Source: CAD feature listing. Evaluate the final solid. Frame: model axes, mm. A direction names the side the tool comes from. Round coordinates to 2 decimals unless told otherwise and drop trailing zeros. Order: outer loops, then holes, each group sorted by start corner. A loop starts at its lowest first (then second) coordinate and runs counter-clockwise, first axis right, second up. Notation, with made-up numbers: (62, 6.5) -> (77, 6.5) arc R29 cw to (77, 44.5) -> close; hole circle Ø4 at (62, 23.25). An arc over 180 degrees is marked (long way). Write item = value, one per line. Start each with the question number.
(1) Reachability of faces 1 (the face through (-26.959, -3.989, 4.068)), 2 (the face through (-102.128, -75, 50)) from +Z, -Z, +X, -X, +Y, -Y: full face, straight path, thin tool, end or side. Return the list, or none.
(2) Ray query, line 1 (X direction, y = -47, z = 56); line 2 (Y direction, x = -47.5, z = 81.5); line 3 (Z direction, x = -49, y = -128). Return the intervals inside material, ascending.
(3) Cut plane B-B on y = -57. Return the cut outline in (x, z).
(4) Cut plane C-C on x = 36. Return the cut outline in (y, z), then the cut area to 3 significant figures.
(5) Cut plane A-A on z = 40. Return the cut outline in (x, y).
from build123d import *

# Parameters (mm, degrees)
F0_W         = 152.4
F0_H         = 101.6
F1_DEPTH     = 152.4
F2_T         = -2.54
F3_T1_DEPTH  = 147.32
F3_T3_DEPTH  = 147.32
F3_T5_DEPTH  = 147.32
F3_T7_DEPTH  = 147.32
F3_T13_DEPTH = 160.02
F3_T19_DEPTH = 160.02
F3_T28_DEPTH = 160.02
F3_T34_DEPTH = 160.02
F3_T43_DEPTH = 160.02
F3_T49_DEPTH = 160.02
F3_T58_DEPTH = 160.02
F3_T64_DEPTH = 160.02


# Not quite as in the source:
# - a fillet or chamfer that OpenCascade refuses, or shapes differently, is made with other operations: its cross-section is extruded or revolved along the edge and cut away or added


with BuildPart() as f1:
    # F0 (on Front) → F1 (new body)
    with BuildSketch(Plane.XZ):
        with Locations((-25.9277992306, 50.8)):
            Rectangle(F0_W, F0_H)
    extrude(amount=F1_DEPTH)

    # F2
    f2_openings = [f1.faces().sort_by_distance(p)[0] for p in [
        (-25.927799, -76.2, 101.6),
    ]]
    offset(amount=F2_T, openings=f2_openings)

    # F3: fillet of radius 5.08 on 8 edges, made by hand

    # F3_s2 → F3_t1 (join)
    with BuildSketch(Plane.XZ.offset(2.54)):
        with BuildLine():
            ThreePointArc((47.7322007694, 7.62), (46.2443032178, 4.0278975516), (42.6522007694, 2.54))
            Line((42.6522007694, 2.54), (47.7322007694, 2.54))
            Line((47.7322007694, 2.54), (47.7322007694, 7.62))
        make_face()
        with BuildLine():
            ThreePointArc((-99.5877992306, 7.62), (-98.0999016791, 4.0278975516), (-94.5077992306, 2.54))
            Line((-94.5077992306, 2.54), (-99.5877992306, 2.54))
            Line((-99.5877992306, 2.54), (-99.5877992306, 7.62))
        make_face()
    extrude(amount=F3_T1_DEPTH)

    # F3_s4 → F3_t3 (join)
    with BuildSketch(Plane.YZ.offset(-99.5877992306)):
        with BuildLine():
            ThreePointArc((-2.54, 7.62), (-4.0278975516, 4.0278975516), (-7.62, 2.54))
            Line((-7.62, 2.54), (-2.54, 2.54))
            Line((-2.54, 2.54), (-2.54, 7.62))
        make_face()
        with BuildLine():
            ThreePointArc((-149.86, 7.62), (-148.3721024484, 4.0278975516), (-144.78, 2.54))
            Line((-144.78, 2.54), (-149.86, 2.54))
            Line((-149.86, 2.54), (-149.86, 7.62))
        make_face()
    extrude(amount=F3_T3_DEPTH)

    # F3_s6 → F3_t5 (cut)
    with BuildSketch(Plane.YZ.offset(-99.5877992306)):
        with BuildLine():
            ThreePointArc((2.54, 101.6), (-1.0521024484, 100.1121024484), (-2.54, 96.52))
            Line((-2.54, 96.52), (-2.54, 101.6))
            Line((-2.54, 101.6), (2.54, 101.6))
        make_face()
        with BuildLine():
            ThreePointArc((-154.94, 101.6), (-151.3478975516, 100.1121024484), (-149.86, 96.52))
            Line((-149.86, 96.52), (-149.86, 101.6))
            Line((-149.86, 101.6), (-154.94, 101.6))
        make_face()
    extrude(amount=F3_T5_DEPTH, mode=Mode.SUBTRACT)

    # F3_s8 → F3_t7 (cut)
    with BuildSketch(Plane.XZ.offset(2.54)):
        with BuildLine():
            ThreePointArc((52.8122007694, 101.6), (49.2200983209, 100.1121024484), (47.7322007694, 96.52))
            Line((47.7322007694, 96.52), (47.7322007694, 101.6))
            Line((47.7322007694, 101.6), (52.8122007694, 101.6))
        make_face()
        with BuildLine():
            ThreePointArc((-104.6677992306, 101.6), (-101.0756967822, 100.1121024484), (-99.5877992306, 96.52))
            Line((-99.5877992306, 96.52), (-99.5877992306, 101.6))
            Line((-99.5877992306, 101.6), (-104.6677992306, 101.6))
        make_face()
    extrude(amount=F3_T7_DEPTH, mode=Mode.SUBTRACT)


with BuildPart() as f3_tool11:
    # F3_s12 → F3_t13 (new body)
    with BuildSketch(Plane.XZ.offset(-10.16)):
        with BuildLine():
            ThreePointArc((52.8122007694, 101.6), (49.2200983209, 100.1121024484), (47.7322007694, 96.52))
            Line((47.7322007694, 96.52), (47.7322007694, 101.6))
            Line((47.7322007694, 101.6), (52.8122007694, 101.6))
        make_face()
    extrude(amount=F3_T13_DEPTH)

    split(bisect_by=Plane.XZ, keep=Keep.TOP)

    split(bisect_by=Plane.YZ.offset(50.2722007694), keep=Keep.BOTTOM)

    split(bisect_by=Plane.XZ.offset(2.54), keep=Keep.BOTTOM)


with BuildPart() as f3_tool17:
    # F3_s18 → F3_t19 (new body)
    with BuildSketch(Plane.YZ.offset(60.4322007694)):
        with BuildLine():
            ThreePointArc((2.54, 101.6), (-1.0521024484, 100.1121024484), (-2.54, 96.52))
            Line((-2.54, 96.52), (-2.54, 101.6))
            Line((-2.54, 101.6), (2.54, 101.6))
        make_face()
    extrude(amount=-F3_T19_DEPTH)

    split(bisect_by=Plane.XZ, keep=Keep.TOP)

    split(bisect_by=Plane.YZ.offset(50.2722007694), keep=Keep.BOTTOM)

    split(bisect_by=Plane.YZ.offset(47.7322007694), keep=Keep.TOP)


with BuildPart() as f3_tool11_1:
    add(f3_tool11.part)

    # F3_t23: intersect F3_tool17
    add(f3_tool17.part, mode=Mode.INTERSECT)


with BuildPart() as f1_1:
    add(f1.part)

    # F3_t9: cut F3_tool11
    add(f3_tool11_1.part, mode=Mode.SUBTRACT)


with BuildPart() as f3_tool26:
    # F3_s27 → F3_t28 (new body)
    with BuildSketch(Plane.YZ.offset(47.7322007694)):
        with BuildLine():
            ThreePointArc((2.54, 101.6), (-1.0521024484, 100.1121024484), (-2.54, 96.52))
            Line((-2.54, 96.52), (-2.54, 101.6))
            Line((-2.54, 101.6), (2.54, 101.6))
        make_face()
    extrude(amount=-F3_T28_DEPTH)

    split(bisect_by=Plane.YZ.offset(-102.1277992306), keep=Keep.TOP)

    split(bisect_by=Plane.XZ, keep=Keep.TOP)

    split(bisect_by=Plane.YZ.offset(-99.5877992306), keep=Keep.BOTTOM)


with BuildPart() as f3_tool32:
    # F3_s33 → F3_t34 (new body)
    with BuildSketch(Plane.XZ.offset(-10.16)):
        with BuildLine():
            ThreePointArc((-104.6677992306, 101.6), (-101.0756967822, 100.1121024484), (-99.5877992306, 96.52))
            Line((-99.5877992306, 96.52), (-99.5877992306, 101.6))
            Line((-99.5877992306, 101.6), (-104.6677992306, 101.6))
        make_face()
    extrude(amount=F3_T34_DEPTH)

    split(bisect_by=Plane.YZ.offset(-102.1277992306), keep=Keep.TOP)

    split(bisect_by=Plane.XZ, keep=Keep.TOP)

    split(bisect_by=Plane.XZ.offset(2.54), keep=Keep.BOTTOM)


with BuildPart() as f3_tool26_1:
    add(f3_tool26.part)

    # F3_t38: intersect F3_tool32
    add(f3_tool32.part, mode=Mode.INTERSECT)


with BuildPart() as f1_2:
    add(f1_1.part)

    # F3_t24: cut F3_tool26
    add(f3_tool26_1.part, mode=Mode.SUBTRACT)


with BuildPart() as f3_tool41:
    # F3_s42 → F3_t43 (new body)
    with BuildSketch(Plane.XZ.offset(2.54)):
        with BuildLine():
            ThreePointArc((52.8122007694, 101.6), (49.2200983209, 100.1121024484), (47.7322007694, 96.52))
            Line((47.7322007694, 96.52), (47.7322007694, 101.6))
            Line((47.7322007694, 101.6), (52.8122007694, 101.6))
        make_face()
    extrude(amount=F3_T43_DEPTH)

    split(bisect_by=Plane.XZ.offset(152.4), keep=Keep.BOTTOM)

    split(bisect_by=Plane.YZ.offset(50.2722007694), keep=Keep.BOTTOM)

    split(bisect_by=Plane.XZ.offset(149.86), keep=Keep.TOP)


with BuildPart() as f3_tool47:
    # F3_s48 → F3_t49 (new body)
    with BuildSketch(Plane.YZ.offset(60.4322007694)):
        with BuildLine():
            ThreePointArc((-154.94, 101.6), (-151.3478975516, 100.1121024484), (-149.86, 96.52))
            Line((-149.86, 96.52), (-149.86, 101.6))
            Line((-149.86, 101.6), (-154.94, 101.6))
        make_face()
    extrude(amount=-F3_T49_DEPTH)

    split(bisect_by=Plane.XZ.offset(152.4), keep=Keep.BOTTOM)

    split(bisect_by=Plane.YZ.offset(50.2722007694), keep=Keep.BOTTOM)

    split(bisect_by=Plane.YZ.offset(47.7322007694), keep=Keep.TOP)


with BuildPart() as f3_tool41_1:
    add(f3_tool41.part)

    # F3_t53: intersect F3_tool47
    add(f3_tool47.part, mode=Mode.INTERSECT)


with BuildPart() as f1_3:
    add(f1_2.part)

    # F3_t39: cut F3_tool41
    add(f3_tool41_1.part, mode=Mode.SUBTRACT)


with BuildPart() as f3_tool56:
    # F3_s57 → F3_t58 (new body)
    with BuildSketch(Plane.XZ.offset(2.54)):
        with BuildLine():
            ThreePointArc((-104.6677992306, 101.6), (-101.0756967822, 100.1121024484), (-99.5877992306, 96.52))
            Line((-99.5877992306, 96.52), (-99.5877992306, 101.6))
            Line((-99.5877992306, 101.6), (-104.6677992306, 101.6))
        make_face()
    extrude(amount=F3_T58_DEPTH)

    split(bisect_by=Plane.YZ.offset(-102.1277992306), keep=Keep.TOP)

    split(bisect_by=Plane.XZ.offset(152.4), keep=Keep.BOTTOM)

    split(bisect_by=Plane.XZ.offset(149.86), keep=Keep.TOP)


with BuildPart() as f3_tool62:
    # F3_s63 → F3_t64 (new body)
    with BuildSketch(Plane.YZ.offset(47.7322007694)):
        with BuildLine():
            ThreePointArc((-154.94, 101.6), (-151.3478975516, 100.1121024484), (-149.86, 96.52))
            Line((-149.86, 96.52), (-149.86, 101.6))
            Line((-149.86, 101.6), (-154.94, 101.6))
        make_face()
    extrude(amount=-F3_T64_DEPTH)

    split(bisect_by=Plane.YZ.offset(-102.1277992306), keep=Keep.TOP)

    split(bisect_by=Plane.XZ.offset(152.4), keep=Keep.BOTTOM)

    split(bisect_by=Plane.YZ.offset(-99.5877992306), keep=Keep.BOTTOM)


with BuildPart() as f3_tool56_1:
    add(f3_tool56.part)

    # F3_t68: intersect F3_tool62
    add(f3_tool62.part, mode=Mode.INTERSECT)


with BuildPart() as f1_4:
    add(f1_3.part)

    # F3_t54: cut F3_tool56
    add(f3_tool56_1.part, mode=Mode.SUBTRACT)


solid = f1_4.part
Evaluation:
q1.face_1 = +Z
q1.face_2 = +Z, -Z, -X, +Y, -Y
q2.line_1 = -102.13 to -99.59, 47.73 to 50.27
q2.line_2 = -152.4 to -149.86, -2.54 to 0
q2.line_3 = 0 to 2.54
q3.outline = (-102.13, 0) -> (50.27, 0) -> (50.27, 100.92) arc R5.08 ccw to (47.73, 96.52) -> (47.73, 7.62) arc R5.08 cw to (42.65, 2.54) -> (-94.51, 2.54) arc R5.08 cw to (-99.59, 7.62) -> (-99.59, 96.52) arc R5.08 ccw to (-102.13, 100.92) -> close
q4.outline = (-152.4, 0) -> (0, 0) -> (0, 100.92) arc R5.08 ccw to (-2.54, 96.52) -> (-2.54, 7.62) arc R5.08 cw to (-7.62, 2.54) -> (-144.78, 2.54) arc R5.08 cw to (-149.86, 7.62) -> (-149.86, 96.52) arc R5.08 ccw to (-152.4, 100.92) -> close
q4.area = 891 mm^2
q5.outline = (-102.13, -152.4) -> (50.27, -152.4) -> (50.27, 0) -> (-102.13, 0) -> close; hole (-99.59, -149.86) -> (47.73, -149.86) -> (47.73, -2.54) -> (-99.59, -2.54) -> close
